Here's how the part is built. I have some questions about the finished solid (model axes, mm). Round coordinates to 2 decimals unless told otherwise and drop trailing zeros. Order: outer loops, then holes, each group sorted by start corner. A loop starts at its lowest first (then second) coordinate and runs counter-clockwise, first axis right, second up. Notation, with made-up numbers: (49, 80) - (107, 80) arc R13 ccw to (107, 104) - close; hole circle Ø11 at (-13, 47). An arc over 180 degrees is marked (long way). One line per item, written item: value.
from build123d import *

# Parameters (mm, degrees)
SKETCH1_R           = 4
SKETCH1_R_2         = 1.5
BOSS_EXTRUDE1_DEPTH = 5
CUT_EXTRUDE1_REACH  = 7
SKETCH2_R           = 11
SKETCH3_W           = 21
SKETCH3_H           = 5
CUT_EXTRUDE2_DEPTH  = 7


with BuildPart() as part:
    # Sketch1 → Boss-Extrude1 (new body)
    with BuildSketch(Plane(origin=(0, 0, 0), x_dir=(1, 0, 0), z_dir=(0, 1, 0))):
        Polygon((-50, 44), (-30, 44), (-30, 49), (-10, 49), (-10, 44), (10, 44), (10, 49), (30, 49), (30, 44), (50, 44), (50, -31), (-50, -31), align=None)
        Circle(SKETCH1_R, mode=Mode.SUBTRACT)
        with Locations((15.5, 15.5)):
            Circle(SKETCH1_R_2, mode=Mode.SUBTRACT)
        with Locations((-15.5, 15.5)):
            Circle(SKETCH1_R_2, mode=Mode.SUBTRACT)
        with Locations((-15.5, -15.5)):
            Circle(SKETCH1_R_2, mode=Mode.SUBTRACT)
        with Locations((15.5, -15.5)):
            Circle(SKETCH1_R_2, mode=Mode.SUBTRACT)
        with Locations((-25, -11)):
            Circle(SKETCH1_R, mode=Mode.SUBTRACT)
        with Locations((25, -11)):
            Circle(SKETCH1_R, mode=Mode.SUBTRACT)
    extrude(amount=BOSS_EXTRUDE1_DEPTH)

    # Sketch2 → Cut-Extrude1 (cut, up to next)
    with BuildSketch(Plane(origin=(0, 5, 0), x_dir=(1, 0, 0), z_dir=(0, 1, 0)), mode=Mode.PRIVATE) as cut_extrude1_sk1:
        Circle(SKETCH2_R)
    cut_extrude1_tool1 = extrude(cut_extrude1_sk1.sketch, amount=-CUT_EXTRUDE1_REACH, mode=Mode.PRIVATE) & part.part
    add(cut_extrude1_tool1.solids().sort_by_distance((0, 5, 0))[0], mode=Mode.SUBTRACT)

    # Sketch3 → Cut-Extrude2 (cut)
    with BuildSketch(Plane(origin=(50, 0, 0), x_dir=(0, 0, -1), z_dir=(1, 0, 0))):
        with Locations((-20.5, 2.5)):
            Rectangle(SKETCH3_W, SKETCH3_H)
    extrude(amount=-CUT_EXTRUDE2_DEPTH, mode=Mode.SUBTRACT)


solid = part.part
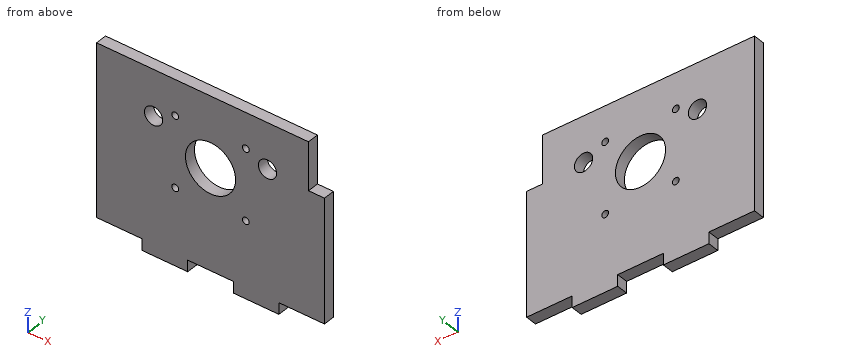
Q1. If I drill on line 1 along X through (y, z) = (1.7, -15.5); line 2 along X through (y, z) = (3.35, 0); line 3 along Z through (x, y) = (25, 3.25), over which ranges is the centre line in solid material (lowest first)?
Results list:
line 1: -50 to -17, -14 to 14, 17 to 50
line 2: -50 to -11, 11 to 50
line 3: -49 to 7, 15 to 31
Q2. Will these pins go through, and if not, where does the flat tip stop? pin 1 (1.5 mm diameter, centred on x = -1, y = 3, fed in from -Z); pin 2 (5 mm diameter, centred on x = 15.5, z = 15.5, fed in from -Y); pin 3 (1.5 mm diameter, centred on y = 3.5, z = -47, fed in from +X); pin 4 (1.5 mm diameter, centred on y = 2, z = 23.5, fed in from +X).
Results list:
pin 1: z = -44
pin 2: y = 0
pin 3: x = 30
pin 4: x = 43
Q3. If we section it at D-D, the plane z = 3.5: Please give me the cut outline in (x, y).
Results list:
outline: (-50, 0) - (-10.43, 0) - (-10.43, 5) - (-50, 5) - close; (10.43, 0) - (50, 0) - (50, 5) - (10.43, 5) - close
Q4. If we section it at C-C, the plane x = -25: Please give me the cut outline in (y, z).
Results list:
outline: (0, -49) - (5, -49) - (5, 7) - (0, 7) - close; (0, 15) - (5, 15) - (5, 31) - (0, 31) - close
Q5. If we section it at B-B, the plane z = -15.5: Please give me the cut outline in (x, y), then the cut area to 3 significant figures.
Results list:
outline: (-50, 0) - (-17, 0) - (-17, 5) - (-50, 5) - close; (-14, 0) - (14, 0) - (14, 5) - (-14, 5) - close; (17, 0) - (50, 0) - (50, 5) - (17, 5) - close
area: 470 mm²
Q6. If we section it at A-A, the plane y = 4.1: Please give me the cut outline in (x, z), then the cut area to 3 significant figures.
Results list:
outline: (-50, -44) - (-30, -44) - (-30, -49) - (-10, -49) - (-10, -44) - (10, -44) - (10, -49) - (30, -49) - (30, -44) - (50, -44) - (50, 10) - (43, 10) - (43, 31) - (-50, 31) - close; hole circle Ø8 at (-25, 11); hole circle Ø3 at (-15.5, -15.5); hole circle Ø3 at (-15.5, 15.5); hole circle Ø22 at (0, 0); hole circle Ø3 at (15.5, -15.5); hole circle Ø3 at (15.5, 15.5); hole circle Ø8 at (25, 11)
area: 7,040 mm²
